Verification items for the finished model (mm, model axes). A direction names the side the tool comes from. Round coordinates to 2 decimals unless told otherwise and drop trailing zeros. Write each loop counter-clockwise with the first axis right and the second up, starting at its lowest first coordinate (ties: lowest second). Pieces come first, ordered by that corner, then holes. Notation, with made-up numbers: (-25, 20.25) -> (17, 20.25) arc R6 ccw to (17, 27.25) -> close; hole circle Ø2 at (-3, -37). An arc over 180 degrees is marked (long way). Use CSV: the item, a comma, the result in double quotes.
```python
from build123d import *

# Parameters (mm, degrees)
F1_DEPTH = 6
F2_R     = 0.3


with BuildPart() as f1:
    # F0 (on Top) → F1 (new body)
    with BuildSketch(Plane.XY):
        with BuildLine():
            Line((-3.5, 0.5), (-3.5, -0.5))
            Line((-3.5, -0.5), (-1.4142135624, -0.5))
            ThreePointArc((-1.4142135624, -0.5), (-1.5, 0), (-1.4142135624, 0.5))
            Line((-1.4142135624, 0.5), (-3.5, 0.5))
        make_face()
        with BuildLine():
            ThreePointArc((-1.4142135624, 0.5), (-1.5, 0), (-1.4142135624, -0.5))
            Line((-1.4142135624, -0.5), (-0.9233092656, -0.5))
            ThreePointArc((-0.9233092656, -0.5), (-1.05, 0), (-0.9233092656, 0.5))
            Line((-0.9233092656, 0.5), (-1.4142135624, 0.5))
        make_face()
        with BuildLine():
            Line((-0.9233092656, -0.5), (-1.4142135624, -0.5))
            ThreePointArc((-1.4142135624, -0.5), (0, -1.5), (1.4142135624, -0.5))
            Line((1.4142135624, -0.5), (0.9233092656, -0.5))
            ThreePointArc((0.9233092656, -0.5), (0, -1.05), (-0.9233092656, -0.5))
        make_face()
        with BuildLine():
            ThreePointArc((1.4142135624, 0.5), (0, 1.5), (-1.4142135624, 0.5))
            Line((-1.4142135624, 0.5), (-0.9233092656, 0.5))
            ThreePointArc((-0.9233092656, 0.5), (0, 1.05), (0.9233092656, 0.5))
            Line((0.9233092656, 0.5), (1.4142135624, 0.5))
        make_face()
        with BuildLine():
            ThreePointArc((1.5, 0), (1.4783978395, -0.2536529681), (1.4142135624, -0.5))
            Line((1.4142135624, -0.5), (3.5, -0.5))
            Line((3.5, -0.5), (3.5, 0.5))
            Line((3.5, 0.5), (1.4142135624, 0.5))
            ThreePointArc((1.4142135624, 0.5), (1.4783978395, 0.2536529681), (1.5, 0))
        make_face()
        with BuildLine():
            Line((0.9233092656, -0.5), (1.4142135624, -0.5))
            ThreePointArc((1.4142135624, -0.5), (1.4783978395, -0.2536529681), (1.5, 0))
            ThreePointArc((1.5, 0), (1.4783978395, 0.2536529681), (1.4142135624, 0.5))
            Line((1.4142135624, 0.5), (0.9233092656, 0.5))
            ThreePointArc((0.9233092656, 0.5), (1.0178346449, 0.2579004373), (1.05, 0))
            ThreePointArc((1.05, 0), (1.0178346449, -0.2579004373), (0.9233092656, -0.5))
        make_face()
    extrude(amount=F1_DEPTH)

    # F2
    f2_edges = [f1.edges().sort_by_distance(p)[0] for p in [
        (1.414214, -0.5, 3),
        (-1.414214, -0.5, 3),
        (1.414214, 0.5, 3),
        (-1.414214, 0.5, 3),
    ]]
    fillet(f2_edges, radius=F2_R)


solid = f1.part
```
Q1. Section check B-B (z = 1.75). Record the cut outline in (x, y).
Filled in:
outline,"(-3.5, -0.5) -> (-1.61, -0.5) arc R0.3 cw to (-1.34, -0.67) arc R1.5 ccw to (1.34, -0.67) arc R0.3 cw to (1.61, -0.5) -> (3.5, -0.5) -> (3.5, 0.5) -> (1.61, 0.5) arc R0.3 cw to (1.34, 0.67) arc R1.5 ccw to (-1.34, 0.67) arc R0.3 cw to (-1.61, 0.5) -> (-3.5, 0.5) -> close; hole circle Ø2.1 at (0, 0)"
Q2. Section check D-D (x = -2.5). Record the cut outline in (y, z).
Filled in:
outline,"(-0.5, 0) -> (0.5, 0) -> (0.5, 6) -> (-0.5, 6) -> close"
Q3. Material ranges on L1, parallel to Y at x = -3, z = 1.6; L2, parallel to X at y = 0.9, z = 0.45; L3, parallel to Y at x = -0.5, z = 0.65, recorded low to high.
Filled in:
L1,"-0.5 to 0.5"
L2,"-1.2 to -0.54, 0.54 to 1.2"
L3,"-1.41 to -0.92, 0.92 to 1.41"
Q4. Go/stop test with flat-tipped pins: P1, Ø1.5, axis at x = 2.5, z = 3, coming from the +Y side; P2, Ø0.9, axis at x = 2.5, z = 4.5, coming from the -Y side. Record where each tip stops, or that it passes through.
Filled in:
P1,"y = 0.5"
P2,"y = -0.5"
Q5. Section check A-A (x = 0.5). Record the cut outline in (y, z).
Filled in:
outline,"(-1.41, 0) -> (-0.92, 0) -> (-0.92, 6) -> (-1.41, 6) -> close; (0.92, 0) -> (1.41, 0) -> (1.41, 6) -> (0.92, 6) -> close"
Q6. Section check C-C (y = 0.4). Record the cut outline in (x, z).
Filled in:
outline,"(-3.5, 0) -> (-0.97, 0) -> (-0.97, 6) -> (-3.5, 6) -> close; (0.97, 0) -> (3.5, 0) -> (3.5, 6) -> (0.97, 6) -> close"
Q7. Access from +Z, -Z, +X, -X, +Y, -Y to the whole of each face (thin tool, end or side, straight path). Record for faces 1 (the flat face through (-3, 0.5, 3)), 2 (the flat face through (-3, -0.5, 3)), 3 (the flat face through (3, -0.5, 3)), 4 (the flat face through (3, 0.5, 3)).
Filled in:
face 1,"+Z, -Z, -X, +Y"
face 2,"+Z, -Z, -X, -Y"
face 3,"+Z, -Z, +X, -Y"
face 4,"+Z, -Z, +X, +Y"
